CAD build for the part. Positions are in the model's coordinates, mm. Face numbers are marked on the shaded views. Coordinates: 2 decimals unless noted, no trailing zeros. Write each loop counter-clockwise with the first axis right and the second up, starting at its lowest first coordinate (ties: lowest second). Pieces come first, ordered by that corner, then holes. Notation, with made-up numbers: (67.5, 86) - (110.5, 86) arc R9 ccw to (110.5, 91) - close; hole circle Ø2 at (-39.5, 80.5). An arc over 180 degrees is marked (long way). Answer in a Markdown table with one row per item. Add a question column.
Q1. Band-saw the part on B-B (y = 20). List the corners of the cut face in (x, z).
Q2. Band-saw the part on D-D (z = 3.25). State how many separate pieces and enclosed holes the cut face has, and give its area (3 significant figures).
Q3. Drill centre lines: line 1 along Y through (x, z) = (95.25, 2.75); line 2 along X through (y, z) = (25.4, 1.35); line 3 along Y through (x, z) = (64.5, 5). Where is each one in solid material? Low to high. Write a range as from..to.
Q4. Two-plate mould, pull along X, no slides. Class the marked faces 1 and 2: +X half, -X half, draft (parallel to the pull), parting line (faces both ways), or undercut.
Q5. Band-saw the part on A-A (x = 42). List the corners of the cut face in (y, z).
Q6. Pin check, flat tips, straight feed: pin 1 (4 mm diameter, centred on x = 19.5, y = 25, fed in from -Z); pin 2 (4.5 mm diameter, centred on x = 6.35, y = 6.35, fed in from -Z); pin 3 (4.5 mm diameter, centred on x = 76.2, y = 25.4, fed in from +Z); pin 4 (1.4 mm diameter, centred on x = 75.5, y = 26.5, fed in from -Z). Stop position of each tip, or through.
Q7. Band-saw the part on C-C (x = 6.35). List the corners of the cut face in (y, z), and give its area (3 significant figures).
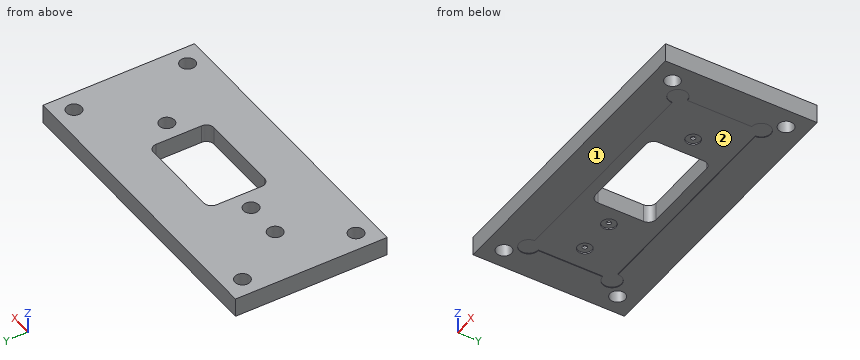
```python
from build123d import *

# Parameters (mm, degrees)
F0_W      = 101.6
F0_H      = 50.8
F1_DEPTH  = 6.35
F3_DEPTH  = 0.254
F4_R      = 2.54
F5_DEPTH  = 6.351
F6_R      = 2.38125
F7_DEPTH  = 0.508
F8_R      = 0.79375
F9_DEPTH  = 1.27
F10_R     = 2.54
F11_DEPTH = 4.826
F13_DEPTH = 6.096


# Not quite as in the source:
# - a feature names something its author has since deleted; it is built from what else it names


with BuildPart() as f1:
    # F0 (on Top) → F1 (new body)
    with BuildSketch(Plane.XY):
        with Locations((50.8, 25.4)):
            Rectangle(F0_W, F0_H)
    extrude(amount=F1_DEPTH)

    # F2 (on face) → F3 (cut)
    with BuildSketch(Plane(origin=(0, 0, 0), x_dir=(1, 0, 0), z_dir=(0, 0, -1))):
        with BuildLine():
            Line((11.43, -14.605), (11.43, -11.43))
            Line((11.43, -11.43), (14.605, -11.43))
            ThreePointArc((14.605, -11.43), (9.1849359697, -9.1849359697), (11.43, -14.605))
        make_face()
        with BuildLine():
            Line((14.605, -11.43), (11.43, -11.43))
            Line((11.43, -11.43), (11.43, -14.605))
            ThreePointArc((11.43, -14.605), (13.6750640303, -13.6750640303), (14.605, -11.43))
        make_face()
        with BuildLine():
            Line((86.995, -11.43), (14.605, -11.43))
            ThreePointArc((14.605, -11.43), (13.6750640303, -13.6750640303), (11.43, -14.605))
            Line((11.43, -14.605), (11.43, -36.195))
            ThreePointArc((11.43, -36.195), (13.6750640303, -37.1249359697), (14.605, -39.37))
            Line((14.605, -39.37), (86.995, -39.37))
            ThreePointArc((86.995, -39.37), (87.9249359697, -37.1249359697), (90.17, -36.195))
            Line((90.17, -36.195), (90.17, -14.605))
            ThreePointArc((90.17, -14.605), (87.9249359697, -13.6750640303), (86.995, -11.43))
        make_face()
        with BuildLine():
            ThreePointArc((93.345, -11.43), (90.17, -8.255), (86.995, -11.43))
            Line((86.995, -11.43), (90.17, -11.43))
            Line((90.17, -11.43), (90.17, -14.605))
            ThreePointArc((90.17, -14.605), (92.4150640303, -13.6750640303), (93.345, -11.43))
        make_face()
        with BuildLine():
            Line((90.17, -11.43), (86.995, -11.43))
            ThreePointArc((86.995, -11.43), (87.9249359697, -13.6750640303), (90.17, -14.605))
            Line((90.17, -14.605), (90.17, -11.43))
        make_face()
        with BuildLine():
            ThreePointArc((14.605, -39.37), (13.6750640303, -37.1249359697), (11.43, -36.195))
            Line((11.43, -36.195), (11.43, -39.37))
            Line((11.43, -39.37), (14.605, -39.37))
        make_face()
        with BuildLine():
            Line((11.43, -39.37), (11.43, -36.195))
            ThreePointArc((11.43, -36.195), (9.1849359697, -41.6150640303), (14.605, -39.37))
            Line((14.605, -39.37), (11.43, -39.37))
        make_face()
        with BuildLine():
            ThreePointArc((93.345, -39.37), (92.4150640303, -37.1249359697), (90.17, -36.195))
            Line((90.17, -36.195), (90.17, -39.37))
            Line((90.17, -39.37), (86.995, -39.37))
            ThreePointArc((86.995, -39.37), (90.17, -42.545), (93.345, -39.37))
        make_face()
        with BuildLine():
            Line((90.17, -39.37), (90.17, -36.195))
            ThreePointArc((90.17, -36.195), (87.9249359697, -37.1249359697), (86.995, -39.37))
            Line((86.995, -39.37), (90.17, -39.37))
        make_face()
    extrude(amount=-F3_DEPTH, mode=Mode.SUBTRACT)

    # F4 (on face) → F5 (cut, through all)
    with BuildSketch(Plane(origin=(0, 0, 0), x_dir=(1, 0, 0), z_dir=(0, 0, -1))):
        with Locations((95.25, -6.35)):
            Circle(F4_R)
        with Locations((6.35, -6.35)):
            Circle(F4_R)
        with Locations((6.35, -44.45)):
            Circle(F4_R)
        with Locations((95.25, -44.45)):
            Circle(F4_R)
    extrude(amount=-F5_DEPTH, mode=Mode.SUBTRACT)

    # F6 (on face) → F7 (cut)
    with BuildSketch(Plane(origin=(0, 0, 0.254), x_dir=(1, 0, 0), z_dir=(0, 0, -1))):
        with Locations((31.75, -25.4)):
            Circle(F6_R)
        with Locations((19.05, -25.4)):
            Circle(F6_R)
        with Locations((76.2, -25.4)):
            Circle(F6_R)
    extrude(amount=-F7_DEPTH, mode=Mode.SUBTRACT)

    # F8 (on face) → F9 (cut)
    with BuildSketch(Plane(origin=(0, 0, 0.762), x_dir=(1, 0, 0), z_dir=(0, 0, -1))):
        with Locations((19.05, -25.4)):
            Circle(F8_R)
        with Locations((31.75, -25.4)):
            Circle(F8_R)
        with Locations((76.2, -25.4)):
            Circle(F8_R)
    extrude(amount=-F9_DEPTH, mode=Mode.SUBTRACT)

    # F10 (on face) → F11 (cut)
    with BuildSketch(Plane.XY.offset(6.35)):
        with Locations((19.05, 25.4)):
            Circle(F10_R)
        with Locations((31.75, 25.4)):
            Circle(F10_R)
        with Locations((76.2, 25.4)):
            Circle(F10_R)
    extrude(amount=-F11_DEPTH, mode=Mode.SUBTRACT)

    # F12 (on face) → F13 (cut, through all)
    with BuildSketch(Plane(origin=(0, 0, 0.254), x_dir=(1, 0, 0), z_dir=(0, 0, -1))):
        with BuildLine():
            Line((67.31, -15.24), (40.64, -15.24))
            ThreePointArc((40.64, -15.24), (38.8439487758, -15.9839487758), (38.1, -17.78))
            Line((38.1, -17.78), (38.1, -33.02))
            ThreePointArc((38.1, -33.02), (38.8439487758, -34.8160512242), (40.64, -35.56))
            Line((40.64, -35.56), (67.31, -35.56))
            ThreePointArc((67.31, -35.56), (69.1060512242, -34.8160512242), (69.85, -33.02))
            Line((69.85, -33.02), (69.85, -17.78))
            ThreePointArc((69.85, -17.78), (69.1060512242, -15.9839487758), (67.31, -15.24))
        make_face()
    extrude(amount=-F13_DEPTH, mode=Mode.SUBTRACT)


solid = f1.part
```
Checked values:
| question | item | result |
|---|---|---|
| 1 | outline | (0, 0) - (11.43, 0) - (11.43, 0.25) - (38.1, 0.25) - (38.1, 6.35) - (0, 6.35) - close; (69.85, 0.25) - (90.17, 0.25) - (90.17, 0) - (101.6, 0) - (101.6, 6.35) - (69.85, 6.35) - close |
| 2 | separate pieces | 1 |
| 2 | enclosed holes | 8 |
| 2 | area | 4,380 mm² |
| 3 | line 1 | y = 0..3.81, 8.89..41.91, 46.99..50.8 |
| 3 | line 2 | x = 0..18.26, 19.84..30.96, 32.54..38.1, 69.85..75.41, 76.99..101.6 |
| 3 | line 3 | y = 0..15.24, 35.56..50.8 |
| 4 | face 1 | draft |
| 4 | face 2 | undercut |
| 5 | outline | (0, 0) - (11.43, 0) - (11.43, 0.25) - (15.24, 0.25) - (15.24, 6.35) - (0, 6.35) - close; (35.56, 0.25) - (39.37, 0.25) - (39.37, 0) - (50.8, 0) - (50.8, 6.35) - (35.56, 6.35) - close |
| 6 | pin 1 | stops at z = 0.25 |
| 6 | pin 2 | passes through |
| 6 | pin 3 | stops at z = 1.52 |
| 6 | pin 4 | stops at z = 0.76 |
| 7 | outline | (0, 0) - (3.81, 0) - (3.81, 6.35) - (0, 6.35) - close; (8.89, 0) - (41.91, 0) - (41.91, 6.35) - (8.89, 6.35) - close; (46.99, 0) - (50.8, 0) - (50.8, 6.35) - (46.99, 6.35) - close |
| 7 | area | 258 mm² |
